Check sheet for the modelled part. Datum: model origin and axes. Units: mm. A direction names the side the tool comes from. Round coordinates to 2 decimals unless told otherwise and drop trailing zeros. Write each loop counter-clockwise with the first axis right and the second up, starting at its lowest first coordinate (ties: lowest second). Pieces come first, ordered by that corner, then holes. Notation, with made-up numbers: (34.5, 67) -> (89.5, 67) arc R21 cw to (89.5, 102) -> close; hole circle Ø9 at (21, -23.5). An arc over 180 degrees is marked (long way). Use one line per item in the form item = value. Start each with the question number.
```python
from build123d import *

# Parameters (mm, degrees)
SKETCH1_W           = 86.36
SKETCH1_H           = 63.5
BOSS_EXTRUDE1_DEPTH = 19.05
CUT_EXTRUDE1_DEPTH  = 63.5
SKETCH3_W           = 14.224
SKETCH3_H           = 46.228
CUT_EXTRUDE4_DEPTH  = 63.5
SKETCH4_R           = 2.032
CUT_EXTRUDE5_DEPTH  = 63.5
SKETCH6_W           = 48
SKETCH6_H           = 55
CUT_EXTRUDE6_DEPTH  = 17
SKETCH7_W           = 15
SKETCH7_H           = 10
CUT_EXTRUDE10_DEPTH = 17
SKETCH9_W           = 26
SKETCH9_H           = 20
CUT_EXTRUDE11_DEPTH = 10
SKETCH10_W          = 52.188826159
SKETCH10_H          = 6.083943305
CUT_EXTRUDE12_DEPTH = 5


with BuildPart() as part:
    # Sketch1 → Boss-Extrude1 (new body)
    with BuildSketch(Plane(origin=(0, 0, 0), x_dir=(1, 0, 0), z_dir=(0, 1, 0))):
        Rectangle(SKETCH1_W, SKETCH1_H)
    extrude(amount=BOSS_EXTRUDE1_DEPTH)

    # Sketch2 → Cut-Extrude1 (cut)
    with BuildSketch(Plane.XY.offset(31.75)):
        with BuildLine():
            Line((-43.18, 19.05), (-43.18, 0))
            Line((-43.18, 0), (-33.232925003, 0))
            ThreePointArc((-33.232925003, 0), (-39.877976383, 9.510716436), (-33.274, 19.05))
            Line((-33.274, 19.05), (-43.18, 19.05))
        make_face()
        with BuildLine():
            Line((43.18, 19.05), (43.18, 0))
            Line((43.18, 0), (33.232925003, 0))
            ThreePointArc((33.232925003, 0), (39.877976383, 9.510716436), (33.274, 19.05))
            Line((33.274, 19.05), (43.18, 19.05))
        make_face()
    extrude(amount=-CUT_EXTRUDE1_DEPTH, mode=Mode.SUBTRACT)

    # Sketch3 → Cut-Extrude4 (cut)
    with BuildSketch(Plane(origin=(0, 19.05, 0), x_dir=(1, 0, 0), z_dir=(0, 1, 0))):
        with Locations((-32.766, 0)):
            Rectangle(SKETCH3_W, SKETCH3_H)
        with Locations((32.766, 0)):
            Rectangle(SKETCH3_W, SKETCH3_H)
    extrude(amount=-CUT_EXTRUDE4_DEPTH, mode=Mode.SUBTRACT)

    # Sketch4 → Cut-Extrude5 (cut)
    with BuildSketch(Plane.XY.offset(31.75)):
        with Locations((-31.75, 9.525)):
            Circle(SKETCH4_R)
        with Locations((31.75, 9.525)):
            Circle(SKETCH4_R)
    extrude(amount=-CUT_EXTRUDE5_DEPTH, mode=Mode.SUBTRACT)

    # Sketch6 → Cut-Extrude6 (cut)
    with BuildSketch(Plane(origin=(0, 19.05, 0), x_dir=(1, 0, 0), z_dir=(0, 1, 0))):
        Rectangle(SKETCH6_W, SKETCH6_H)
    extrude(amount=-CUT_EXTRUDE6_DEPTH, mode=Mode.SUBTRACT)

    # Sketch7 → Cut-Extrude10 (cut)
    with BuildSketch(Plane(origin=(25.654, 0, 0), x_dir=(0, 0, -1), z_dir=(1, 0, 0))):
        with Locations((-10.886, 7.2)):
            Rectangle(SKETCH7_W, SKETCH7_H)
    extrude(amount=-CUT_EXTRUDE10_DEPTH, mode=Mode.SUBTRACT)

    # Sketch9 → Cut-Extrude11 (cut)
    with BuildSketch(Plane(origin=(0, 0, -31.75), x_dir=(-1, 0, 0), z_dir=(0, 0, -1))):
        Rectangle(SKETCH9_W, SKETCH9_H)
    extrude(amount=-CUT_EXTRUDE11_DEPTH, mode=Mode.SUBTRACT)

    # Sketch10 → Cut-Extrude12 (cut)
    with BuildSketch(Plane.XY.offset(31.75)):
        with Locations((0.33271565, 6.150312699)):
            Rectangle(SKETCH10_W, SKETCH10_H)
    extrude(amount=-CUT_EXTRUDE12_DEPTH, mode=Mode.SUBTRACT)


solid = part.part
```
1. Sectioned sample at D-D (z = -24). Enter the section's corners in (x, y) (3 decimals).
2. Scan lines: probe 1 along Z at (x, y) = (-23, 17.75); probe 2 along X at (y, z) = (13.25, -13); probe 3 along Y at (x, z) = (31.75, 28.5). Record each from-to range of solid material in increasing order.
3. Sectioned sample at B-B (z = 11.5). Enter the section's corners in (x, y), and give its area (3 significant figures).
4. Sectioned sample at A-A (x = 14.5). Enter the section's corners in (y, z), and give its area (3 significant figures).
5. Depth check by flat-ended pin: pin 1 (5.5 mm diameter, centred on y = 8, z = -3.5, fed in from +X); pin 2 (1.3 mm diameter, centred on x = 25, y = 7.5, fed in from +Z); pin 3 (2.5 mm diameter, centred on y = 6.5, z = 29, fed in from -X). Enter the tip coordinate at first touch or a pass-through.
6. Tool access check on faces 1 (the face through (0, 13, -27.5)), 2 (the face through (-13, 4, -29)), 3 (the face through (-32.9, 7.5, 23.114)), 4 (the face through (32.7, 7.5, 23.114)). Record the directions out of +Z, -Z, +X, -X, +Y, -Y that give a thin tool (end or side, any length) a straight path to the whole face; none if there is none.
7. Sectioned sample at C-C (x = 31.75). Enter the section's corners in (y, z).
8. Mould release check, pull along X, two halves, no side actions. Record for faces 5 (the face through (39.876, 9.338, 27.492)), 6 (the face through (-39.876, 9.338, -27.372)), 7 (the face through (0, 3.108, 30)), 8 (the face through (-25, 19.05, 0)): +X half, -X half, draft (parallel to the pull), parting line (faces both ways), or undercut.
Returned:
q1.outline = (-33.274, 19.05) arc R10.16 ccw to (-33.233, 0) -> (-13, 0) -> (-13, 2.05) -> (-24, 2.05) -> (-24, 19.05) -> close; (13, 0) -> (33.233, 0) arc R10.16 ccw to (33.274, 19.05) -> (24, 19.05) -> (24, 2.05) -> (13, 2.05) -> close; hole circle Ø4.064 at (-31.75, 9.525); hole circle Ø4.064 at (31.75, 9.525)
q2.probe_1 = -31.75 to -27.5, 27.5 to 31.75
q2.probe_2 = -25.65 to -24, 24 to 25.65
q2.probe_3 = 0 to 7.49, 11.56 to 19.05
q3.outline = (-25.65, 0) -> (25.65, 0) -> (25.65, 2.2) -> (24, 2.2) -> (24, 2.05) -> (-24, 2.05) -> (-24, 19.05) -> (-25.65, 19.05) -> close; (24, 12.2) -> (25.65, 12.2) -> (25.65, 19.05) -> (24, 19.05) -> close
q3.area = 145 mm^2
q4.outline = (0, -31.75) -> (19.05, -31.75) -> (19.05, -27.5) -> (2.05, -27.5) -> (2.05, 27.5) -> (3.11, 27.5) -> (3.11, 31.75) -> (0, 31.75) -> close; (9.19, 27.5) -> (19.05, 27.5) -> (19.05, 31.75) -> (9.19, 31.75) -> close
q4.area = 249 mm^2
q5.pin_1 = 25.65
q5.pin_2 = 26.75
q5.pin_3 = -39.72
q6.face_1 = +Y
q6.face_2 = -Z, -Y
q6.face_3 = -X, +Y, -Y
q6.face_4 = +X, +Y, -Y
q7.outline = (0, -31.75) -> (7.49, -31.75) -> (7.49, -23.11) -> (0, -23.11) -> close; (0, 23.11) -> (7.49, 23.11) -> (7.49, 31.75) -> (0, 31.75) -> close; (11.56, -31.75) -> (19.05, -31.75) -> (19.05, -23.11) -> (11.56, -23.11) -> close; (11.56, 23.11) -> (19.05, 23.11) -> (19.05, 31.75) -> (11.56, 31.75) -> close
q8.face_5 = +X half
q8.face_6 = -X half
q8.face_7 = undercut
q8.face_8 = draft
